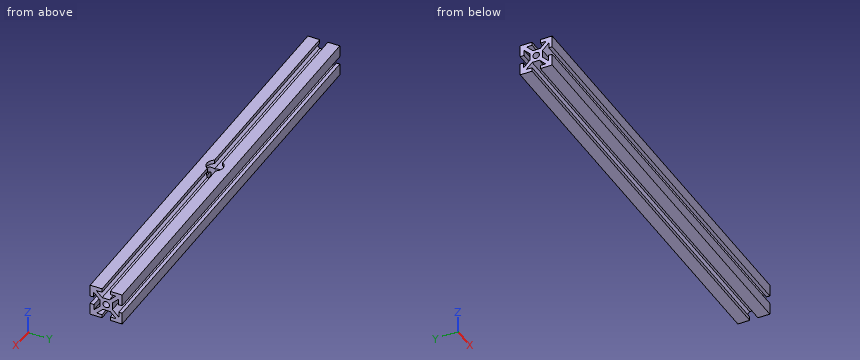
from build123d import *

# Parameters (mm, degrees)
SKETCH1_W           = 10
SKETCH1_H           = 10
SKETCH1_R           = 2.605
BOSS_EXTRUDE1_DEPTH = 330.2
CIRPATTERN1_COUNT   = 4
SKETCH2_R           = 6.35
CUT_EXTRUDE1_DEPTH  = 20


with BuildPart() as part:
    # Sketch1 → Boss-Extrude1 (new body)
    with BuildSketch(Plane(origin=(0, 0, 0), x_dir=(0, 0, -1), z_dir=(1, 0, 0))):
        Rectangle(SKETCH1_W, SKETCH1_H)
        Circle(SKETCH1_R, mode=Mode.SUBTRACT)
        Polygon((7.474873734, 9.921463197), (2.553410537, 5), (5, 5), (5, 3.203948776), (9.596194078, 7.800142853), align=None)
        Polygon((9.596194078, 3.24), (12.596194078, 3.24), (12.596194078, 12.596194078), (3.24, 12.596194078), (3.24, 9.921463197), (7.474873734, 9.921463197), (9.596194078, 7.800142853), align=None)
    boss_extrude1 = extrude(amount=BOSS_EXTRUDE1_DEPTH)

    # CirPattern1: Boss-Extrude1 ×4 about axis
    cirpattern1_axis = Axis((0, 0, 0), (1, 0, 0))
    for i in range(1, CIRPATTERN1_COUNT):
        add(boss_extrude1.rotate(cirpattern1_axis, i * 360 / CIRPATTERN1_COUNT))

    # Sketch2 → Cut-Extrude1 (cut)
    with BuildSketch(Plane.XY):
        with Locations((165.1, 0)):
            Circle(SKETCH2_R)
    extrude(amount=CUT_EXTRUDE1_DEPTH, mode=Mode.SUBTRACT)


solid = part.part
The listing builds one solid part. Answer for the finished solid, in the listing's coordinates (mm). Round coordinates to 2 decimals unless told otherwise and drop trailing zeros. Answer in a Markdown table with one row per item. Add a question column.
1) Consider line 1 along Y through (x, z) = (173.5, -10.5); line 2 along Y through (x, z) = (254.5, 0) (3 decimals). Determine where each line is inside the solid, lowest interval first. Write a range as from..to.
2) Flat-ended cylindrical pins translate along their axes: pin 1 Ø6 at (x, y) = (176, 2) entering from +Z; pin 2 Ø1.7 at (x, z) = (213, -1) entering from -Y; pin 3 Ø2.5 at (x, y) = (167, 4) entering from +Z. Find the tip coordinate at first contact, or state that the pin passes through.
3) The part is cut by section A-A on x = 165.1. Count the separate pieces of the cut face and the enclosed holes in it, plus the area to 3 significant figures.
Findings below:
| question | item | result |
|---|---|---|
| 1 | line 1 | y = -12.6..-3.24, 3.24..12.6 |
| 1 | line 2 | y = -5..-2.605, 2.605..5 |
| 2 | pin 1 | stops at z = 12.6 |
| 2 | pin 2 | stops at y = -5 |
| 2 | pin 3 | stops at z = 0 |
| 3 | separate pieces | 3 |
| 3 | enclosed holes | 0 |
| 3 | area | 267 mm² |
